from build123d import *

# Parameters (mm, degrees)
F1_DEPTH = 150
F3_DEPTH = 15
F3_TAPER = -45


with BuildPart() as f1:
    # F0 (on Front) → F1 (new body)
    with BuildSketch(Plane.XZ):
        Polygon((16.4764662622, 10.6293191202), (-16.6578079225, 10.6293191202), (-16.4379915805, 3.9366264828), (-3.308858315, 3.9366264828), (-3.308858315, -18.7284196727), (3.3802918042, -18.7284196727), (3.3802918042, 4.1624740697), (16.4764662622, 4.1624740697), align=None)
    extrude(amount=F1_DEPTH)

    # F2 (on face) → F3 (join)
    with BuildSketch(Plane(origin=(0, 0, 0), x_dir=(-1, 0, 0), z_dir=(0, 1, 0))):
        Polygon((16.4379915805, 3.9366264828), (16.6578079225, 10.6293191202), (-16.4764662622, 10.6293191202), (-16.4764662622, 4.1624740697), (-3.3802918042, 4.1624740697), (-3.3802918042, -18.7284196727), (3.308858315, -18.7284196727), (3.308858315, 3.9366264828), align=None)
    extrude(amount=F3_DEPTH, taper=F3_TAPER)


solid = f1.part
Work out the finished part from the listing and answer in its coordinate system (mm). A direction names the side the tool comes from. Give positions to 0.01 mm unless a question says otherwise; leave off trailing zeros. Write each loop counter-clockwise with the first axis right and the second up, starting at its lowest first coordinate (ties: lowest second). Pieces come first, ordered by that corner, then holes.
Q1. A tool of negligible diameter and unlimited length cuts with its end or side. For faces 1 (the face through (-10, -74, 3.937)), 2 (the face through (3.38, -74, -7)), 3 (the face through (0, -74, 10.629)), from which of +Z, -Z, +X, -X, +Y, -Y can it reach the whole face along a straight path? Write none if from no direction.
Answer:
face 1: -Z, -X, -Y
face 2: -Z, +X, -Y
face 3: +Z, +X, -X, -Y
Q2. Given pin 1 (25 mm diameter, centred on y = -43.5, z = -6, fed in from +X); pin 2 (11.5 mm diameter, centred on y = -54, z = -7, fed in from -X); pin 3 (5.5 mm diameter, centred on x = 1.5, y = -48, fed in from -Z), each flat-ended and moving along its own axis, determine where each tip first touches the part or whether it passes through.
Answer:
pin 1: stops at x = 16.48
pin 2: stops at x = -3.31
pin 3: stops at z = -18.73
Q3. The part is cut by section A-A on y = -82.5. Give the vertices of the cut face in (x, z), and give its area (3 significant figures).
Answer:
outline: (-16.66, 10.63) - (-16.44, 3.94) - (-3.31, 3.94) - (-3.31, -18.73) - (3.38, -18.73) - (3.38, 4.16) - (16.48, 4.16) - (16.48, 10.63) - close
area: 370 mm2
Q4. Straight lines are drawn through the part: L1, parallel to X at y = -89.5, z = -4.5; L2, parallel to X at y = -67, z = 5; L3, parallel to Z at x = -12, y = -28. For each, find the intervals that lie inside material, in ascending order.
Answer:
L1: x = -3.31 to 3.38
L2: x = -16.47 to 16.48
L3: z = 3.94 to 10.63
